Read the model definition and answer for the solid it produces. Units are mm, in the model's axes. Coordinates: 2 decimals unless noted, no trailing zeros. Order: outer loops, then holes, each group sorted by start corner. A loop starts at its lowest first (then second) coordinate and runs counter-clockwise, first axis right, second up. Notation, with made-up numbers: M 5,22.25 L 47,22.25 A19 ccw 47,56.25 Z; hole C 18,76 d10. An arc over 180 degrees is marked long. Put each result on its own line as item: value.
from build123d import *

# Parameters (mm, degrees)
MODEL_R             = 1.6
BOSS_EXTRUDE1_DEPTH = 3


with BuildPart() as part:
    # Model → Boss-Extrude1 (new body)
    with BuildSketch(Plane.XY):
        with BuildLine():
            Line((-70.5, 76.5), (-70.5, 70))
            ThreePointArc((-70.5, 70), (-71.378679656, 67.878679656), (-73.5, 67))
            Line((-73.5, 67), (-74, 67))
            ThreePointArc((-74, 67), (-78, 63), (-74, 59))
            Line((-74, 59), (-73.5, 59))
            ThreePointArc((-73.5, 59), (-71.378679656, 58.121320344), (-70.5, 56))
            Line((-70.5, 56), (-70.5, -56))
            ThreePointArc((-70.5, -56), (-71.378679656, -58.121320344), (-73.5, -59))
            Line((-73.5, -59), (-74, -59))
            ThreePointArc((-74, -59), (-78, -63), (-74, -67))
            Line((-74, -67), (-73.5, -67))
            ThreePointArc((-73.5, -67), (-71.378679656, -67.878679656), (-70.5, -70))
            Line((-70.5, -70), (-70.5, -76.5))
            ThreePointArc((-70.5, -76.5), (-69.328427125, -79.328427125), (-66.5, -80.5))
            Line((-66.5, -80.5), (66.5, -80.5))
            ThreePointArc((66.5, -80.5), (69.328427125, -79.328427125), (70.5, -76.5))
            Line((70.5, -76.5), (70.5, -70))
            ThreePointArc((70.5, -70), (71.378679656, -67.878679656), (73.5, -67))
            Line((73.5, -67), (74, -67))
            ThreePointArc((74, -67), (78, -63), (74, -59))
            Line((74, -59), (73.5, -59))
            ThreePointArc((73.5, -59), (71.378679656, -58.121320344), (70.5, -56))
            Line((70.5, -56), (70.5, 56))
            ThreePointArc((70.5, 56), (71.378679656, 58.121320344), (73.5, 59))
            Line((73.5, 59), (74, 59))
            ThreePointArc((74, 59), (78, 63), (74, 67))
            Line((74, 67), (73.5, 67))
            ThreePointArc((73.5, 67), (71.378679656, 67.878679656), (70.5, 70))
            Line((70.5, 70), (70.5, 76.5))
            ThreePointArc((70.5, 76.5), (69.328427125, 79.328427125), (66.5, 80.5))
            Line((66.5, 80.5), (-66.5, 80.5))
            ThreePointArc((-66.5, 80.5), (-69.328427125, 79.328427125), (-70.5, 76.5))
        make_face()
        with Locations((66.5, 76.5)):
            Circle(MODEL_R, mode=Mode.SUBTRACT)
        with Locations((66.5, -76.5)):
            Circle(MODEL_R, mode=Mode.SUBTRACT)
        with Locations((-66.5, 76.5)):
            Circle(MODEL_R, mode=Mode.SUBTRACT)
        with Locations((-66.5, -76.5)):
            Circle(MODEL_R, mode=Mode.SUBTRACT)
        with Locations((-74, 63)):
            Circle(MODEL_R, mode=Mode.SUBTRACT)
        with Locations((74, 63)):
            Circle(MODEL_R, mode=Mode.SUBTRACT)
        with Locations((-74, -63)):
            Circle(MODEL_R, mode=Mode.SUBTRACT)
        with Locations((74, -63)):
            Circle(MODEL_R, mode=Mode.SUBTRACT)
        with Locations((29, -53)):
            Circle(MODEL_R, mode=Mode.SUBTRACT)
        with Locations((29, -4)):
            Circle(MODEL_R, mode=Mode.SUBTRACT)
        with Locations((-29, -53)):
            Circle(MODEL_R, mode=Mode.SUBTRACT)
        with Locations((-29, -4)):
            Circle(MODEL_R, mode=Mode.SUBTRACT)
        with Locations((29, 76.5)):
            Circle(MODEL_R, mode=Mode.SUBTRACT)
        with Locations((-29, 76.5)):
            Circle(MODEL_R, mode=Mode.SUBTRACT)
        with BuildLine():
            Line((-62.5, 69.5), (-62.5, -69.5))
            ThreePointArc((-62.5, -69.5), (-61.621320344, -71.621320344), (-59.5, -72.5))
            Line((-59.5, -72.5), (-36, -72.5))
            ThreePointArc((-36, -72.5), (-33.878679656, -71.621320344), (-33, -69.5))
            Line((-33, -69.5), (-33, 69.5))
            ThreePointArc((-33, 69.5), (-33.878679656, 71.621320344), (-36, 72.5))
            Line((-36, 72.5), (-59.5, 72.5))
            ThreePointArc((-59.5, 72.5), (-61.621320344, 71.621320344), (-62.5, 69.5))
        make_face(mode=Mode.SUBTRACT)
        with BuildLine():
            Line((-22, -72.5), (22, -72.5))
            ThreePointArc((22, -72.5), (24.121320344, -71.621320344), (25, -69.5))
            Line((25, -69.5), (25, -60))
            ThreePointArc((25, -60), (24.121320344, -57.878679656), (22, -57))
            Line((22, -57), (-22, -57))
            ThreePointArc((-22, -57), (-24.121320344, -57.878679656), (-25, -60))
            Line((-25, -60), (-25, -69.5))
            ThreePointArc((-25, -69.5), (-24.121320344, -71.621320344), (-22, -72.5))
        make_face(mode=Mode.SUBTRACT)
        with BuildLine():
            Line((36, -72.5), (59.5, -72.5))
            ThreePointArc((59.5, -72.5), (61.621320344, -71.621320344), (62.5, -69.5))
            Line((62.5, -69.5), (62.5, 69.5))
            ThreePointArc((62.5, 69.5), (61.621320344, 71.621320344), (59.5, 72.5))
            Line((59.5, 72.5), (36, 72.5))
            ThreePointArc((36, 72.5), (33.878679656, 71.621320344), (33, 69.5))
            Line((33, 69.5), (33, -69.5))
            ThreePointArc((33, -69.5), (33.878679656, -71.621320344), (36, -72.5))
        make_face(mode=Mode.SUBTRACT)
        with BuildLine():
            Line((22, 72.5), (-22, 72.5))
            ThreePointArc((-22, 72.5), (-24.121320344, 71.621320344), (-25, 69.5))
            Line((-25, 69.5), (-25, 3))
            ThreePointArc((-25, 3), (-24.121320344, 0.878679656), (-22, 0))
            Line((-22, 0), (22, 0))
            ThreePointArc((22, 0), (24.121320344, 0.878679656), (25, 3))
            Line((25, 3), (25, 69.5))
            ThreePointArc((25, 69.5), (24.121320344, 71.621320344), (22, 72.5))
        make_face(mode=Mode.SUBTRACT)
        with BuildLine():
            Line((-25, -11), (-25, -46))
            ThreePointArc((-25, -46), (-24.121320344, -48.121320344), (-22, -49))
            Line((-22, -49), (22, -49))
            ThreePointArc((22, -49), (24.121320344, -48.121320344), (25, -46))
            Line((25, -46), (25, -11))
            ThreePointArc((25, -11), (24.121320344, -8.878679656), (22, -8))
            Line((22, -8), (-22, -8))
            ThreePointArc((-22, -8), (-24.121320344, -8.878679656), (-25, -11))
        make_face(mode=Mode.SUBTRACT)
    extrude(amount=BOSS_EXTRUDE1_DEPTH)


solid = part.part
Q1. For a pull along Y with two mould halves and no side action, classify faces 1 (the face through (69.297, -79.359, 1.479)), 2 (the face through (-78, 63, 1)), 3 (the face through (0, -6, 3)) as +Y half, -Y half, draft (parallel to the pull), parting line (faces both ways), or undercut.
Answers below:
face 1: -Y half
face 2: undercut
face 3: draft
Q2. Consider line 1 along X through (y, z) = (76.5, 1.3); line 2 along X through (y, z) = (-76.5, 2.1); line 3 along X through (y, z) = (56.5, 1.65). Determine where each line is inside the solid, lowest interval first.
Answers below:
line 1: x = -70.5 to -68.1, -64.9 to -30.6, -27.4 to 27.4, 30.6 to 64.9, 68.1 to 70.5
line 2: x = -70.5 to -68.1, -64.9 to 64.9, 68.1 to 70.5
line 3: x = -70.54 to -62.5, -33 to -25, 25 to 33, 62.5 to 70.54
Q3. Find section D-D on z = 1.1. Give the number of separate pieces and of enclosed holes in the cut face, plus the area to 3 significant figures.
Answers below:
separate pieces: 1
enclosed holes: 19
area: 7,840 mm^2
Q4. Given pin 1 (1.5 mm diameter, centred on y = 2, z = 1.5, fed in from -X); pin 2 (0.9 mm diameter, centred on y = 73.5, z = 1, fed in from +X); pin 3 (1.5 mm diameter, centred on y = -65, z = 1.5, fed in from +X); pin 4 (5 mm diameter, centred on x = 29, y = 76.5, fed in from +Z), each flat-ended and moving along its own axis, determine where each tip first touches the part or whether it passes through.
Answers below:
pin 1: stops at x = -70.5
pin 2: stops at x = 70.5
pin 3: stops at x = 77.8
pin 4: stops at z = 3
Q5. Find section C-C on x = -7.5. Write down the section's boundary in (y, z), plus the area to 3 significant figures.
Answers below:
outline: M -80.5,0 L -72.5,0 L -72.5,3 L -80.5,3 Z; M -57,0 L -49,0 L -49,3 L -57,3 Z; M -8,0 L 0,0 L 0,3 L -8,3 Z; M 72.5,0 L 80.5,0 L 80.5,3 L 72.5,3 Z
area: 96.0 mm^2
Q6. Find section B-B on y = -43.5. Write down the section's boundary in (x, z).
Answers below:
outline: M -70.5,0 L -62.5,0 L -62.5,3 L -70.5,3 Z; M -33,0 L -25,0 L -25,3 L -33,3 Z; M 25,0 L 33,0 L 33,3 L 25,3 Z; M 62.5,0 L 70.5,0 L 70.5,3 L 62.5,3 Z
Q7. Find section A-A on x = 56.5. Write down the section's boundary in (y, z), plus the area to 3 significant figures.
Answers below:
outline: M -80.5,0 L -72.5,0 L -72.5,3 L -80.5,3 Z; M 72.5,0 L 80.5,0 L 80.5,3 L 72.5,3 Z
area: 48.0 mm^2
